Verification items for the finished model (mm, model axes). A direction names the side the tool comes from. Round coordinates to 2 decimals unless told otherwise and drop trailing zeros. Write each loop counter-clockwise with the first axis right and the second up, starting at its lowest first coordinate (ties: lowest second). Pieces come first, ordered by that corner, then holes. Notation, with made-up numbers: M 30,68.5 L 70,68.5 A15 ccw 70,91.5 Z; hole C 50,44 d10. An arc over 180 degrees is marked long. One line per question, with ' | ' between items. Start each with the question number.
Q1. Thickness scan on line 1 along X through (y, z) = (10.75, -5.25); line 2 along Z through (x, y) = (12, 10.25); line 3 along Z through (x, y) = (5.75, 4). Record the ranges inside material, lowest first. Write a range as from..to.
Q2. Tool access check on faces 5 (the face through (4.1, 8.1, -2.8)), 6 (the face through (11.956, 10.487, -5.474)), 7 (the face through (4.1, 0, -6.5)). Record the directions out of +Z, -Z, +X, -X, +Y, -Y that give a thin tool (end or side, any length) a straight path to the whole face; none if there is none.
Q3. Cross-section at C-C (z = -1). Record the boundary of the cut face in (x, y).
Q4. Cross-section at B-B (x = 12.5). Record the boundary of the cut face in (y, z).
Q5. Release check for a two-part mould opening along Z. For faces 1 (the face through (15.85, 9, -4)), 2 (the face through (3.599, 8.987, -4.803)), 3 (the face through (6, 5, -7.85)), 4 (the face through (1.5, 4, -4)) record: released by +Z, released by -Z, zero draft, split by the parting line, or undercut.
Q6. Gauge pin test, flat ends, axial feed: pin 1 (0.6 mm diameter, centred on x = 4, z = -4, fed in from -Y); pin 2 (0.9 mm diameter, centred on x = 12.5, z = -4, fed in from +Y); pin 3 (3.5 mm diameter, centred on x = 11.89, z = -3.92, fed in from -Y). Record the tip position at first contact, or that the pin passes through.
Q7. Cross-section at D-D (y = 5). Record the boundary of the cut face in (x, z).
Q8. Cross-section at A-A (y = 1.5). Record the boundary of the cut face in (x, z).
from build123d import *

# Parameters (mm, degrees)
BOSS_EXTRUDE1_DEPTH = 7.85
SKETCH5_W           = 5.3
SKETCH5_H           = 4.85
CUT_EXTRUDE1_DEPTH  = 8.1
SKETCH6_R           = 2.45
SKETCH6_R_2         = 1.55
BOSS_EXTRUDE3_DEPTH = 1.8
SKETCH7_R           = 0.95
CUT_EXTRUDE2_DEPTH  = 1.8


with BuildPart() as part:
    # Sketch2 → Boss-Extrude1 (new body)
    with BuildSketch(Plane.XY):
        Polygon((0, 9.6), (0, 0), (8.3, 0), (15.85, 8.1), (15.85, 9.6), align=None)
    extrude(amount=-BOSS_EXTRUDE1_DEPTH)

    # Sketch5 → Cut-Extrude1 (cut)
    with BuildSketch(Plane.XZ):
        with Locations((4.15, -3.925)):
            Rectangle(SKETCH5_W, SKETCH5_H)
    extrude(amount=-CUT_EXTRUDE1_DEPTH, mode=Mode.SUBTRACT)

    # Sketch6 → Boss-Extrude3 (add)
    # profile 1 of 2: a face of its own
    with BuildSketch(Plane(origin=(0, 9.6, 0), x_dir=(1, 0, 0), z_dir=(0, 1, 0))):
        with Locations(Location((3.9625, 3.925, 0), (0, 0, 270))):
            Circle(SKETCH6_R)
    # profile 2 of 2: a face of its own
    with BuildSketch(Plane(origin=(0, 9.6, 0), x_dir=(1, 0, 0), z_dir=(0, 1, 0))):
        with Locations(Location((11.8875, 3.925, 0), (0, 0, 270))):
            Circle(SKETCH6_R)
        with Locations(Location((11.8875, 3.925, 0), (0, 0, 270))):
            Circle(SKETCH6_R_2, mode=Mode.SUBTRACT)
    extrude(amount=BOSS_EXTRUDE3_DEPTH)

    # Sketch7 → Cut-Extrude2 (cut)
    with BuildSketch(Plane.XZ.offset(-8.1)):
        with Locations(Location((3.9625, -3.925, 0), (0, 0, 270))):
            Circle(SKETCH7_R)
    extrude(amount=-CUT_EXTRUDE2_DEPTH, mode=Mode.SUBTRACT)


solid = part.part
Determined:
1) line 1: x = 1.9..6.02, 9.83..11.08, 12.69..13.95 | line 2: z = -6.37..-5.47, -2.38..-1.48 | line 3: z = -7.85..-6.35, -1.5..0
2) face 5: -Y | face 6: +Y | face 7: +Z, -Z, +X, -X, -Y
3) outline: M 0,0 L 8.3,0 L 15.85,8.1 L 15.85,9.6 L 0,9.6 Z
4) outline: M 4.51,-7.85 L 9.6,-7.85 L 9.6,-6.3 L 11.4,-6.3 L 11.4,-5.35 L 9.6,-5.35 L 9.6,-2.5 L 11.4,-2.5 L 11.4,-1.55 L 9.6,-1.55 L 9.6,0 L 4.51,0 Z
5) face 1: zero draft | face 2: undercut | face 3: released by -Z | face 4: undercut
6) pin 1: stops at y = 9.9 | pin 2: stops at y = 9.6 | pin 3: stops at y = 1.97
7) outline: M 0,-7.85 L 12.96,-7.85 L 12.96,0 L 0,0 Z; hole M 1.5,-6.35 L 6.8,-6.35 L 6.8,-1.5 L 1.5,-1.5 Z
8) outline: M 0,-7.85 L 9.7,-7.85 L 9.7,0 L 0,0 Z; hole M 1.5,-6.35 L 6.8,-6.35 L 6.8,-1.5 L 1.5,-1.5 Z
